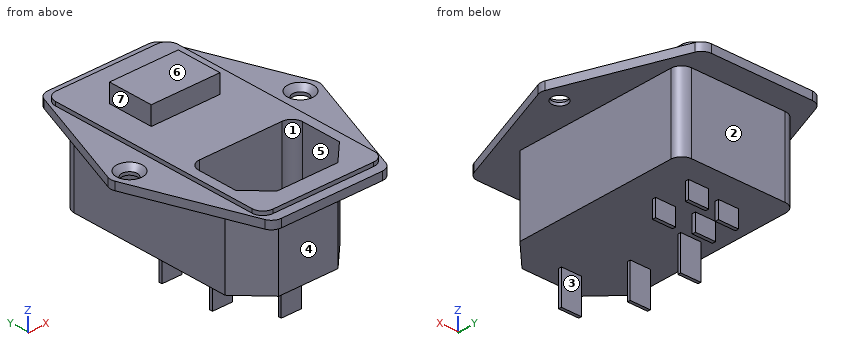
Autodesk Inventor part; units mm, degrees
ref_plane "YZ Plane" through (0, 0, 0) normal (1, 0, 0) x (0, 1, 0)
ref_plane "XZ Plane" through (0, 0, 0) normal (0, 1, 0) x (-1, 0, 0)
ref_plane "XY Plane" through (0, 0, 0) normal (0, 0, 1) x (1, 0, 0)
sketch "Esquisse1" plane through (0, 0, 0) normal (0, 0, 1) x (1, 0, 0)
  line L0 (-13.4, -23.5) -> (13.4, -23.5)
  line L1 (13.4, -23.5) -> (13.4, 23.5)
  line L2 (13.4, 23.5) -> (-13.4, 23.5)
  line L3 (-13.4, 23.5) -> (-13.4, -23.5)
  line L4 (-13.4, -23.5) -> (13.4, 23.5) construction
  line L5 (13.4, -23.5) -> (-13.4, 23.5) construction
  point P0 (0, 0)
  dimension "d0" = 26.8
  dimension "d1" = 47
extrude "Extrusion1" add sketch "Esquisse1" along normal blind 18
chamfer "Chanfrein1" distance 6.5 angle 45 2 edges at (-13.4, -23.5, 9) (13.4, -23.5, 9)
sketch "Esquisse2" plane through (0, 0, 18) normal (0, 0, 1) x (1, 0, 0)
  line L0 (-24.4, 0) -> (-13.5, 29.4)
  line L1 (-13.5, 29.4) -> (13.5, 29.4)
  line L2 (13.5, 29.4) -> (24.4, 0)
  line L3 (24.4, 0) -> (13.5, -29.4)
  line L4 (13.5, -29.4) -> (-13.5, -29.4)
  line L5 (-13.5, -29.4) -> (-24.4, 0)
  point P0 (0, 0)
  point P1 (0, 29.4)
  point P2 (0, -29.4)
  dimension "d7" = 58.8
  dimension "d8" = 29.4
  dimension "d9" = 48.8
  dimension "d10" = 24.4
  dimension "d11" = 27
  dimension "d12" = 27
extrude "Extrusion2" add sketch "Esquisse2" along normal blind 1.9
sketch "Esquisse3" plane through (0, 0, 19.9) normal (0, 0, 1) x (1, 0, 0)
  line L0 (-14.25, -27.25) -> (14.25, -27.25)
  line L1 (14.25, -27.25) -> (14.25, 27.25)
  line L2 (14.25, 27.25) -> (-14.25, 27.25)
  line L3 (-14.25, 27.25) -> (-14.25, -27.25)
  point P0 (0, 0)
  point P1 (-14.25, 0)
  point P2 (0, 27.25)
  dimension "d15" = 28.5
  dimension "d16" = 54.5
extrude "Extrusion3" add sketch "Esquisse3" along normal blind 0.9
sketch "Esquisse4" plane through (0, 0, 20.8) normal (0, 0, 1) x (1, 0, 0)
  line L0 (-7.1, -23.25) -> (7.1, -23.25)
  line L1 (12.1, -18.25) -> (12.1, -9)
  line L2 (9.6, -6.5) -> (-9.6, -6.5)
  line L3 (-12.1, -9) -> (-12.1, -18.25)
  line L4 (-14.25, -27.25) -> (14.25, -27.25)
  line L5 (-7.1, -23.25) -> (-12.1, -18.25)
  line L6 (7.1, -23.25) -> (12.1, -18.25)
  arc A0 (-9.6, -6.5) -> (-12.1, -9) centre (-9.6, -9) ccw
  arc A1 (12.1, -9) -> (9.6, -6.5) centre (9.6, -9) ccw
  point P0 (0, 0)
  point P1 (-12.1, -23.25)
  point P2 (12.1, -23.25)
  point P3 (-12.1, -6.5)
  point P4 (0, -6.5)
  dimension "d19" = 24.2
  dimension "d20" = 16.75
  dimension "d21" = 4
  dimension "d22" = 5
  dimension "d23" = 5
  dimension "d24" = 5
  dimension "d25" = 5
  dimension "d26" = 2.5
extrude "Extrusion4" cut sketch "Esquisse4" against normal blind 18.11
sketch "Esquisse5" plane through (0, 0, 20.8) normal (0, 0, 1) x (1, 0, 0)
  line L0 (-8, 7.4) -> (8, 7.4)
  line L1 (8, 7.4) -> (8, 17.9)
  line L2 (8, 17.9) -> (-8, 17.9)
  line L3 (-8, 17.9) -> (-8, 7.4)
  line L4 (14.25, 27.25) -> (-14.25, 27.25)
  point P0 (0, 0)
  point P1 (0, 7.4)
  dimension "d29" = 16
  dimension "d30" = 10.5
  dimension "d31" = 9.35
extrude "Extrusion5" add sketch "Esquisse5" along normal blind 4.3
sketch "Esquisse6" plane through (0, 0, 0) normal (0, 0, -1) x (-1, 0, 0)
  line L0 (-2.35, -19.2) -> (2.35, -19.2)
  line L1 (2.35, -19.2) -> (2.35, -18.5)
  line L2 (2.35, -18.5) -> (-2.35, -18.5)
  line L3 (-2.35, -18.5) -> (-2.35, -19.2)
  line L4 (4.7, -9.5) -> (9.4, -9.5)
  line L5 (9.4, -9.5) -> (9.4, -8.8)
  line L6 (9.4, -8.8) -> (4.7, -8.8)
  line L7 (4.7, -8.8) -> (4.7, -9.5)
  line L8 (4.7, 3.2) -> (9.4, 3.2)
  line L9 (9.4, 3.2) -> (9.4, 3.9)
  line L10 (9.4, 3.9) -> (4.7, 3.9)
  line L11 (4.7, 3.9) -> (4.7, 3.2)
  line L12 (6.9, -23.5) -> (-6.9, -23.5)
  line L13 (13.4, 23.5) -> (13.4, -17)
  point P0 (0, 0)
  point P1 (0, -19.2)
  dimension "d34" = 4.7
  dimension "d35" = 0.7
  dimension "d38" = 0.7
  dimension "d40" = 0.7
  dimension "d41" = 4.3
  dimension "d42" = 14
  dimension "d43" = 12
  dimension "d44" = 4
  dimension "d45" = 4.7
extrude "Extrusion6" add sketch "Esquisse6" along normal blind 8
sketch "Esquisse7" plane through (0, 0, 0) normal (0, 0, -1) x (-1, 0, 0)
  line L0 (-6.525, 17.2) -> (-1.825, 17.2)
  line L1 (-1.825, 17.2) -> (-1.825, 18)
  line L2 (-1.825, 18) -> (-6.525, 18)
  line L3 (-6.525, 18) -> (-6.525, 17.2)
  line L4 (-6.525, 8.9) -> (-1.825, 8.9)
  line L5 (-1.825, 8.9) -> (-1.825, 9.7)
  line L6 (-1.825, 9.7) -> (-6.525, 9.7)
  line L7 (-6.525, 9.7) -> (-6.525, 8.9)
  line L8 (1.825, 16.5) -> (6.525, 16.5)
  line L9 (6.525, 16.5) -> (6.525, 15.7)
  line L10 (6.525, 15.7) -> (1.825, 15.7)
  line L11 (1.825, 15.7) -> (1.825, 16.5)
  line L12 (1.825, 9.9) -> (6.525, 9.9)
  line L13 (6.525, 9.9) -> (6.525, 10.7)
  line L14 (6.525, 10.7) -> (1.825, 10.7)
  line L15 (1.825, 10.7) -> (1.825, 9.9)
  line L16 (-13.4, 23.5) -> (13.4, 23.5)
  point P0 (0, 0)
  dimension "d48" = 4.7
  dimension "d49" = 4.7
  dimension "d50" = 0.8
  dimension "d51" = 0.8
  dimension "d52" = 0.8
  dimension "d53" = 0.8
  dimension "d54" = 7.5
  dimension "d55" = 5
  dimension "d56" = 3.65
  dimension "d57" = 1.825
  dimension "d58" = 5.5
  dimension "d60" = 1.5
extrude "Extrusion7" add sketch "Esquisse7" along normal blind 4
sketch "Esquisse8" plane through (0, 0, 19.9) normal (0, 0, 1) x (1, 0, 0)
  point P0 (0, 0)
  point P1 (-19.905, 0)
  point P2 (19.905, 0)
  dimension "d63" = 39.81
  dimension "d64" = 19.905
hole "Perçage1" at (-19.905, 0, 19.9) at (19.905, 0, 19.9) direction (0, 0, -1) diameter 3.6 end through all countersink diameter 6 countersink angle 90
fillet "Congé1" radius 2.5 12 edges at (-13.5, 29.4, 18.95) (-13.5, -29.4, 18.95) (13.5, -29.4, 18.95) (13.5, 29.4, 18.95) (24.4, 0, 18.95) (-24.4, 0, 18.95) (-14.25, 27.25, 20.35) (14.25, 27.25, 20.35) (-14.25, -27.25, 20.35) (14.25, -27.25, 20.35) (13.4, 23.5, 9) (-13.4, 23.5, 9)
equation "\"d12\" = d11"
equation "\"d38\" = d35"
equation "\"d40\" = d35"
equation "\"d45\" = d34"
equation "\"d49\" = d48"
equation "\"d51\" = d50"
equation "\"d52\" = d51"
equation "\"d53\" = d52"
equation "\"pi\" = 3.141593"
equation "\"nombredor\" = 1.61803"
properties part number "Plug+prise" material "Plastique ABS"
Work out the finished part from the listing and answer in its coordinate system (mm). Face numbers are marked on the shaded views. A direction names the side the tool comes from. Give positions to 0.01 mm unless a question says otherwise; leave off trailing zeros. Loops run counter-clockwise (first coordinate to the right, second up) from the corner with the lowest first, then second, coordinate; pieces in that order, holes last. Notation, with made-up numbers: (73, 64) -> (120, 64) arc R17 cw to (120, 72) -> close; hole circle Ø7 at (-24, 89.5). An arc over 180 degrees is marked (long way). Use CSV: the item, a comma, the result in double quotes.
1. A tool of negligible diameter and unlimited length cuts with its end or side. For the marked faces 1, 2, 3 and 4, from which of +Z, -Z, +X, -X, +Y, -Y can it reach the whole face along a straight path? Write none if from no direction.
Found:
face 1,"+Z"
face 2,"-Z, +X, -X, +Y"
face 3,"-Z, +X, -X"
face 4,"-Z, +X, -X, -Y"
2. The mould has two halves that part along X. Classify the marked faces 5, 6 and 7: +X half, -X half, draft (parallel to the pull), parting line (faces both ways), or undercut.
Found:
face 5,"undercut"
face 6,"draft"
face 7,"-X half"
3. The part is cut by section D-D (y = -16). Write down the section's boundary in (x, z).
Found:
outline,"(-18.47, 18) -> (-13.4, 18) -> (-13.4, 0) -> (13.4, 0) -> (13.4, 18) -> (18.47, 18) -> (18.47, 19.9) -> (14.25, 19.9) -> (14.25, 20.8) -> (12.1, 20.8) -> (12.1, 2.69) -> (-12.1, 2.69) -> (-12.1, 20.8) -> (-14.25, 20.8) -> (-14.25, 19.9) -> (-18.47, 19.9) -> close"
4. The part is cut by section C-C (z = 1). Write down the section's boundary in (x, y), then the cut area to 3 significant figures.
Found:
outline,"(-13.4, -17) -> (-6.9, -23.5) -> (6.9, -23.5) -> (13.4, -17) -> (13.4, 21) arc R2.5 ccw to (10.9, 23.5) -> (-10.9, 23.5) arc R2.5 ccw to (-13.4, 21) -> close"
area,"1,210 mm^2"
5. The part is cut by section A-A (y = 0). Write down the section's boundary in (x, z) (3 decimals), then the cut area to 3 significant figures.
Found:
outline,"(-24.234, 18) -> (-21.705, 18) -> (-21.705, 18.7) -> (-22.905, 19.9) -> (-24.234, 19.9) -> close; (-18.105, 18) -> (-13.4, 18) -> (-13.4, 0) -> (13.4, 0) -> (13.4, 18) -> (18.105, 18) -> (18.105, 18.7) -> (16.905, 19.9) -> (14.25, 19.9) -> (14.25, 20.8) -> (-14.25, 20.8) -> (-14.25, 19.9) -> (-16.905, 19.9) -> (-18.105, 18.7) -> close; (21.705, 18) -> (24.234, 18) -> (24.234, 19.9) -> (22.905, 19.9) -> (21.705, 18.7) -> close"
area,"584 mm^2"
6. Flat-ended cylindrical pins translate along their axes: pin 1 Ø2 at (y, z) = (20, 12.5) entering from -X; pin 2 Ø2.5 at (x, z) = (-1, -4.5) entering from +Y; pin 3 Ø3 at (x, z) = (1, 13) entering from -Y; pin 4 Ø3 at (x, z) = (18, 16) entering from -Y. Find the tip coordinate at first contact, or state that the pin passes through.
Found:
pin 1,"x = -13.4"
pin 2,"y = 16.5"
pin 3,"y = -23.5"
pin 4,"through"
7. The part is cut by section B-B (z = 10). Write down the section's boundary in (x, y).
Found:
outline,"(-13.4, -17) -> (-6.9, -23.5) -> (6.9, -23.5) -> (13.4, -17) -> (13.4, 21) arc R2.5 ccw to (10.9, 23.5) -> (-10.9, 23.5) arc R2.5 ccw to (-13.4, 21) -> close; hole (-12.1, -18.25) -> (-7.1, -23.25) -> (7.1, -23.25) -> (12.1, -18.25) -> (12.1, -9) arc R2.5 ccw to (9.6, -6.5) -> (-9.6, -6.5) arc R2.5 ccw to (-12.1, -9) -> close"
8. Straight lines are drawn through the part: line 1 (Y direction, x = 5.5, z = 6); line 2 (Y direction, x = 4, z = -0.5); line 3 (Z direction, x = 5, y = 13). For each, find the intervals that lie inside material, in ascending order.
Found:
line 1,"-23.5 to -23.25, -6.5 to 23.5"
line 2,"8.9 to 9.7, 17.2 to 18"
line 3,"0 to 25.1"
